Can you work these out from the model? Positions are in its coordinate system, mm. Face numbers are marked on the shaded views. A direction names the side the tool comes from. Round coordinates to 2 decimals unless told otherwise and drop trailing zeros. Order: outer loops, then holes, each group sorted by start corner. A loop starts at its lowest first (then second) coordinate and runs counter-clockwise, first axis right, second up.
Q1. If I drill on line 1 (X direction, y = 66.5, z = 0); line 2 (X direction, y = 51, z = 11); line 3 (Z direction, x = 4.5, y = 19), over which ranges is the centre line in solid material (lowest first)?
Q2. If we section it at C-C (x = -6): Please give me the cut outline in (y, z).
Q3. For the marked faces 1, 2 and 3, which set-ups out of +Z, -Z, +X, -X, +Y, -Y let a thin tool reach every point of the face, with its end or its side?
Q4. Will these pins go through, and if not, where does the flat tip stop? P1, Ø2, axis at y = 50, z = -17.5, coming from the -X side; P2, Ø1, axis at y = 37.5, z = -18, coming from the -X side; P3, Ø2, axis at y = 97, z = 11, coming from the +X side.
Q5. If we section it at D-D (z = -18): Please give me the cut outline in (x, y).
Q6. If we section it at A-A (y = 88.5): Please give me the cut outline in (x, z), plus the area to 3 significant figures.
Q7. If we section it at B-B (z = 0): Please give me the cut outline in (x, y).
from build123d import *

# Parameters (mm, degrees)
CROQUIS1_R              = 22.5
SALIENTE_EXTRUIR1_DEPTH = 110
CROQUIS2_R              = 16.7
CROQUIS2_R_2            = 13.3
CORTAR_EXTRUIR1_DEPTH   = 90
CROQUIS4_R              = 22.5
CORTAR_EXTRUIR2_DEPTH   = 10
SALIENTE_EXTRUIR2_START = -75
CROQUIS5_R              = 30.5
CROQUIS5_R_2            = 22.5
SALIENTE_EXTRUIR2_DEPTH = 75


with BuildPart() as part:
    # Croquis1 → Saliente-Extruir1 (new body)
    with BuildSketch(Plane(origin=(0, 0, 0), x_dir=(1, 0, 0), z_dir=(0, 1, 0))):
        with Locations(Location((0, 0, 0), (0, 0, 270))):
            Circle(CROQUIS1_R)
    extrude(amount=SALIENTE_EXTRUIR1_DEPTH)

    # Croquis2 → Cortar-Extruir1 (cut)
    with BuildSketch(Plane.XZ):
        with Locations(Location((0, 0, 0), (0, 0, 270))):
            Circle(CROQUIS2_R)
        with Locations(Location((0, 0, 0), (0, 0, 270))):
            Circle(CROQUIS2_R_2, mode=Mode.SUBTRACT)
    extrude(amount=-CORTAR_EXTRUIR1_DEPTH, mode=Mode.SUBTRACT)

    # Croquis4 → Cortar-Extruir2 (cut)
    with BuildSketch(Plane.XZ):
        with Locations(Location((0, 0, 0), (0, 0, 270))):
            Circle(CROQUIS4_R)
    extrude(amount=-CORTAR_EXTRUIR2_DEPTH, mode=Mode.SUBTRACT)

    # Croquis5 → Saliente-Extruir2 (add)
    with BuildSketch(Plane(origin=(0, 100, 0), x_dir=(1, 0, 0), z_dir=(0, 1, 0)).offset(SALIENTE_EXTRUIR2_START)):
        with Locations(Location((0, 0, 0), (0, 0, 270))):
            Circle(CROQUIS5_R)
        with Locations(Location((0, 0, 0), (0, 0, 90))):
            Circle(CROQUIS5_R_2, mode=Mode.SUBTRACT)
    extrude(amount=SALIENTE_EXTRUIR2_DEPTH)


solid = part.part
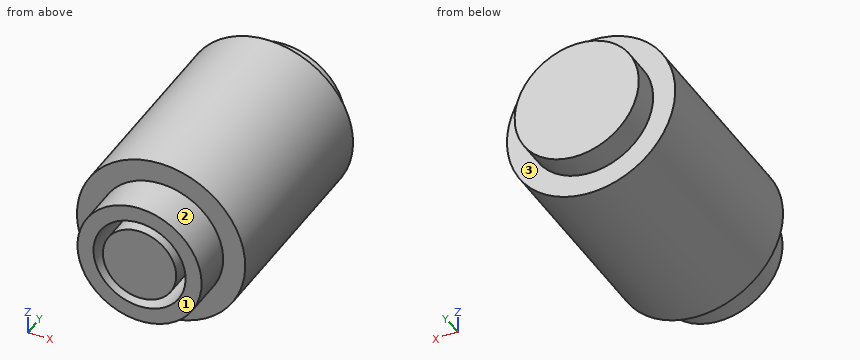
Solution:
1. line 1: x = -30.5 to -16.7, -13.3 to 13.3, 16.7 to 30.5
1. line 2: x = -28.45 to -12.57, -7.48 to 7.48, 12.57 to 28.45
1. line 3: z = -22.05 to -16.08, -12.52 to 12.52, 16.08 to 22.05
2. outline: (10, -21.69) - (25, -21.69) - (25, -29.9) - (100, -29.9) - (100, -21.69) - (110, -21.69) - (110, 21.69) - (100, 21.69) - (100, 29.9) - (25, 29.9) - (25, 21.69) - (10, 21.69) - (10, 15.58) - (90, 15.58) - (90, 11.87) - (10, 11.87) - (10, -11.87) - (90, -11.87) - (90, -15.58) - (10, -15.58) - close
3. face 1: +Z, -Z, +X, -X, -Y
3. face 2: -Y
3. face 3: +Y
4. P1: stops at x = -25.65
4. P2: stops at x = -24.98
4. P3: stops at x = 28.81
5. outline: (-24.62, 25) - (-13.5, 25) - (-13.5, 10) - (13.5, 10) - (13.5, 25) - (24.62, 25) - (24.62, 100) - (13.5, 100) - (13.5, 110) - (-13.5, 110) - (-13.5, 100) - (-24.62, 100) - close
6. outline: circle Ø61 at (0, 0); circle Ø26.6 at (0, 0); hole circle Ø33.4 at (0, 0)
6. area: 2,600 mm2
7. outline: (-30.5, 25) - (-22.5, 25) - (-22.5, 10) - (-16.7, 10) - (-16.7, 90) - (-13.3, 90) - (-13.3, 10) - (13.3, 10) - (13.3, 90) - (16.7, 90) - (16.7, 10) - (22.5, 10) - (22.5, 25) - (30.5, 25) - (30.5, 100) - (22.5, 100) - (22.5, 110) - (-22.5, 110) - (-22.5, 100) - (-30.5, 100) - close
